Part model, mm, in its own coordinate system. A direction names the side the tool comes from. Give positions to 0.01 mm unless a question says otherwise; leave off trailing zeros. Loops run counter-clockwise (first coordinate to the right, second up) from the corner with the lowest first, then second, coordinate; pieces in that order, holes last. Notation, with made-up numbers: M -7.75,64 L 31.25,64 A27 ccw 31.25,99 Z; hole C 0,46.25 d4. An arc over 180 degrees is marked long. Put each result on its own line as item: value. Start each with the question number.
```python
from build123d import *

# Parameters (mm, degrees)
BOSS_EXTRUDE1_DEPTH = 4
SKETCH2_W           = 10
SKETCH2_H           = 4
BOSS_EXTRUDE2_DEPTH = 4
SKETCH3_W           = 4
SKETCH3_H           = 39
BOSS_EXTRUDE3_DEPTH = 4


with BuildPart() as part:
    # Sketch1 → Boss-Extrude1 (new body)
    with BuildSketch(Plane(origin=(0, 0, 0), x_dir=(1, 0, 0), z_dir=(0, 1, 0))):
        Polygon((17.5, 113), (17.5, 114), (27.5, 114), (27.5, -1), (17.5, -1), (17.5, 0), (0, 0), (0, 113), align=None)
    extrude(amount=BOSS_EXTRUDE1_DEPTH)

    # Sketch2 → Boss-Extrude2 (add)
    with BuildSketch(Plane(origin=(0, 4, 0), x_dir=(1, 0, 0), z_dir=(0, 1, 0))):
        with Locations((22.5, -3)):
            Rectangle(SKETCH2_W, SKETCH2_H)
        with Locations((22.5, 116)):
            Rectangle(SKETCH2_W, SKETCH2_H)
    extrude(amount=-BOSS_EXTRUDE2_DEPTH)

    # Sketch3 → Boss-Extrude3 (add)
    with BuildSketch(Plane(origin=(0, 4, 0), x_dir=(1, 0, 0), z_dir=(0, 1, 0))):
        with Locations((29.5, 57.5)):
            Rectangle(SKETCH3_W, SKETCH3_H)
    extrude(amount=-BOSS_EXTRUDE3_DEPTH)


solid = part.part
```
1) Band-saw the part on B-B on x = 13. Give the cut face in (y, z), then the cut area to 3 significant figures.
2) Pin check, flat tips, straight feed: pin 1 Ø2 at (x, y) = (12.5, 2) entering from -Z; pin 2 Ø1.2 at (x, y) = (5, 2) entering from +Z; pin 3 Ø1.2 at (y, z) = (2.5, 3) entering from -X. Stop position of each tip, or through.
3) Which spindle directions (+Z, -Z, +X, -X, +Y, -Y) get a long thin tool onto all of the face, cutting with end or side? Do faces 1 (the flat face through (29, 2, -77)), 2 (the flat face through (9, 2, -113)), 3 (the flat face through (17.5, 2, 3)), 4 (the flat face through (29, 2, -38)). Say none if no direction does.
4) Band-saw the part on A-A on y = 2.75. Give the cut face in (x, z).
5) Wall check: L1, parallel to Z at x = 9.5, y = 3.15; L2, parallel to X at y = 0.9, z = -7.5. Give the ranges that are in metal, low to high.
6) Band-saw the part on C-C on z = -98. Give the cut face in (x, y).
Evaluation:
1. outline: M 0,-113 L 4,-113 L 4,0 L 0,0 Z
1. area: 452 mm2
2. pin 1: z = -113
2. pin 2: z = 0
2. pin 3: x = 17.5
3. face 1: -Z, +X, +Y, -Y
3. face 2: -Z, -X, +Y, -Y
3. face 3: +Z, -X, +Y, -Y
3. face 4: +Z, +X, +Y, -Y
4. outline: M 0,-113 L 17.5,-113 L 17.5,-118 L 27.5,-118 L 27.5,-77 L 31.5,-77 L 31.5,-38 L 27.5,-38 L 27.5,5 L 17.5,5 L 17.5,0 L 0,0 Z
5. L1: -113 to 0
5. L2: 0 to 27.5
6. outline: M 0,0 L 27.5,0 L 27.5,4 L 0,4 Z
